```python
from build123d import *

# Parameters (mm, degrees)
SKETCH_1_W            = 118.4
SKETCH_1_H            = 66.4
EXTRUDE_1_DEPTH       = 5.6
SKETCH_5_R            = 3
CUT_EXTRUDE_961_DEPTH = 3
SKETCH_7_W            = 85
SKETCH_7_H            = 58
LCD_DEPTH             = 3.6
SKETCH_13_W           = 73
SKETCH_13_H           = 46
CUT_EXTRUDE_1_DEPTH   = 10
FILLET_2_R            = 5
FILLET_3_R            = 6


with BuildPart() as part:
    # Эскиз1 → Бобышка-Вытянуть1 (new body)
    with BuildSketch(Plane(origin=(0, 0, 0), x_dir=(1, 0, 0), z_dir=(0, 1, 0))):
        with Locations((-2, 0)):
            Rectangle(SKETCH_1_W, SKETCH_1_H)
    extrude(amount=EXTRUDE_1_DEPTH)

    # Эскиз5 → Cut-Extrude 961 (cut)
    with BuildSketch(Plane.XZ):
        with Locations(Location((-56.16, 21.1, 0), (0, 0, 270))):
            Circle(SKETCH_5_R)
        with Locations(Location((-56.16, -21.9, 0), (0, 0, 90))):
            Circle(SKETCH_5_R)
        with Locations(Location((35.96, 22.3, 0), (0, 0, 270))):
            Circle(SKETCH_5_R)
        with Locations(Location((35.96, -18.7, 0), (0, 0, 90))):
            Circle(SKETCH_5_R)
    extrude(amount=-CUT_EXTRUDE_961_DEPTH, mode=Mode.SUBTRACT)

    # Эскиз7 → под LCD (cut)
    with BuildSketch(Plane.XZ):
        with Locations((-10, 0)):
            Rectangle(SKETCH_7_W, SKETCH_7_H)
    extrude(amount=-LCD_DEPTH, mode=Mode.SUBTRACT)

    # Эскиз13 → Вырез-Вытянуть1 (cut)
    with BuildSketch(Plane.XZ.offset(-3.6)):
        with Locations((-10, 0)):
            Rectangle(SKETCH_13_W, SKETCH_13_H)
    extrude(amount=-CUT_EXTRUDE_1_DEPTH, mode=Mode.SUBTRACT)

    # Скругление2
    # the kernel refuses this fillet: 5 mm, written as the material it takes off along each edge
    with BuildSketch(Plane(origin=(-46.5, 5.6, -23), x_dir=(-1, 0, 0), z_dir=(0, 0, 1)), Plane(origin=(26.5, 5.6, 23), x_dir=(1, 0, 0), z_dir=(0, 0, -1))) as fillet_2_piece_1:
        with BuildLine():
            CenterArc((4, 5), FILLET_2_R, 216.869897646, 53.130102354)
            Line((0, 2), (-0.08, 1.94))
            ThreePointArc((-0.08, 1.94), (-0.1, 1), (-0.1, 0))
            Line((-0.1, 0), (0, -0.1))
            Line((0, -0.1), (4, -0.1))
            Line((4, -0.1), (4, 0))
        make_face()
    extrude(amount=46, mode=Mode.SUBTRACT)
    with BuildSketch(Plane(origin=(-46.5, 5.6, 23), x_dir=(0, 0, 1), z_dir=(1, 0, 0)), Plane(origin=(26.5, 5.6, -23), x_dir=(0, 0, -1), z_dir=(-1, 0, 0))) as fillet_2_piece_2:
        with BuildLine():
            CenterArc((4, 5), FILLET_2_R, 216.869897646, 53.130102354)
            Line((0, 2), (-0.08, 1.94))
            ThreePointArc((-0.08, 1.94), (-0.1, 1), (-0.1, 0))
            Line((-0.1, 0), (0, -0.1))
            Line((0, -0.1), (4, -0.1))
            Line((4, -0.1), (4, 0))
        make_face()
    extrude(amount=73, mode=Mode.SUBTRACT)
    with BuildSketch(Plane(origin=(-46.5, 5.6, -33), x_dir=(-1, 0, 0), z_dir=(0, 0, 1))) as fillet_2_piece_3a_section:
        with BuildLine():
            CenterArc((4, 5), FILLET_2_R, 216.869897646, 53.130102354)
            Line((0, 2), (-0.08, 1.94))
            ThreePointArc((-0.08, 1.94), (-0.1, 1), (-0.1, 0))
            Line((-0.1, 0), (0, -0.1))
            Line((0, -0.1), (4, -0.1))
            Line((4, -0.1), (4, 0))
        make_face()
    fillet_2_piece_3a = extrude(amount=56, mode=Mode.PRIVATE)
    fillet_2_piece_3a = split(fillet_2_piece_3a, bisect_by=Plane(origin=(-47.529417057, 5.088057438, -23), z_dir=(0, 0, -1)), keep=Keep.TOP, mode=Mode.PRIVATE)
    with BuildSketch(Plane(origin=(26.5, 5.6, -23), x_dir=(0, 0, -1), z_dir=(-1, 0, 0))) as fillet_2_piece_3b_section:
        with BuildLine():
            CenterArc((4, 5), FILLET_2_R, 216.869897646, 53.130102354)
            Line((0, 2), (-0.08, 1.94))
            ThreePointArc((-0.08, 1.94), (-0.1, 1), (-0.1, 0))
            Line((-0.1, 0), (0, -0.1))
            Line((0, -0.1), (4, -0.1))
            Line((4, -0.1), (4, 0))
        make_face()
    fillet_2_piece_3b = extrude(amount=83, mode=Mode.PRIVATE)
    fillet_2_piece_3b = split(fillet_2_piece_3b, bisect_by=Plane(origin=(-46.5, 5.088057438, -24.029417057), z_dir=(-1, 0, 0)), keep=Keep.TOP, mode=Mode.PRIVATE)
    fillet_2_piece_3 = fillet_2_piece_3a & fillet_2_piece_3b
    add(fillet_2_piece_3, mode=Mode.SUBTRACT)
    with BuildSketch(Plane(origin=(-46.5, 5.6, -23), x_dir=(-1, 0, 0), z_dir=(0, 0, 1))) as fillet_2_piece_4a_section:
        with BuildLine():
            CenterArc((4, 5), FILLET_2_R, 216.869897646, 53.130102354)
            Line((0, 2), (-0.08, 1.94))
            ThreePointArc((-0.08, 1.94), (-0.1, 1), (-0.1, 0))
            Line((-0.1, 0), (0, -0.1))
            Line((0, -0.1), (4, -0.1))
            Line((4, -0.1), (4, 0))
        make_face()
    fillet_2_piece_4a = extrude(amount=56, mode=Mode.PRIVATE)
    fillet_2_piece_4a = split(fillet_2_piece_4a, bisect_by=Plane(origin=(-47.529417057, 5.088057438, 23), z_dir=(0, 0, 1)), keep=Keep.TOP, mode=Mode.PRIVATE)
    with BuildSketch(Plane(origin=(-56.5, 5.6, 23), x_dir=(0, 0, 1), z_dir=(1, 0, 0))) as fillet_2_piece_4b_section:
        with BuildLine():
            CenterArc((4, 5), FILLET_2_R, 216.869897646, 53.130102354)
            Line((0, 2), (-0.08, 1.94))
            ThreePointArc((-0.08, 1.94), (-0.1, 1), (-0.1, 0))
            Line((-0.1, 0), (0, -0.1))
            Line((0, -0.1), (4, -0.1))
            Line((4, -0.1), (4, 0))
        make_face()
    fillet_2_piece_4b = extrude(amount=83, mode=Mode.PRIVATE)
    fillet_2_piece_4b = split(fillet_2_piece_4b, bisect_by=Plane(origin=(-46.5, 5.088057438, 24.029417057), z_dir=(-1, 0, 0)), keep=Keep.TOP, mode=Mode.PRIVATE)
    fillet_2_piece_4 = fillet_2_piece_4a & fillet_2_piece_4b
    add(fillet_2_piece_4, mode=Mode.SUBTRACT)
    with BuildSketch(Plane(origin=(26.5, 5.6, 33), x_dir=(1, 0, 0), z_dir=(0, 0, -1))) as fillet_2_piece_5a_section:
        with BuildLine():
            CenterArc((4, 5), FILLET_2_R, 216.869897646, 53.130102354)
            Line((0, 2), (-0.08, 1.94))
            ThreePointArc((-0.08, 1.94), (-0.1, 1), (-0.1, 0))
            Line((-0.1, 0), (0, -0.1))
            Line((0, -0.1), (4, -0.1))
            Line((4, -0.1), (4, 0))
        make_face()
    fillet_2_piece_5a = extrude(amount=56, mode=Mode.PRIVATE)
    fillet_2_piece_5a = split(fillet_2_piece_5a, bisect_by=Plane(origin=(27.529417057, 5.088057438, 23), z_dir=(0, 0, 1)), keep=Keep.TOP, mode=Mode.PRIVATE)
    with BuildSketch(Plane(origin=(-46.5, 5.6, 23), x_dir=(0, 0, 1), z_dir=(1, 0, 0))) as fillet_2_piece_5b_section:
        with BuildLine():
            CenterArc((4, 5), FILLET_2_R, 216.869897646, 53.130102354)
            Line((0, 2), (-0.08, 1.94))
            ThreePointArc((-0.08, 1.94), (-0.1, 1), (-0.1, 0))
            Line((-0.1, 0), (0, -0.1))
            Line((0, -0.1), (4, -0.1))
            Line((4, -0.1), (4, 0))
        make_face()
    fillet_2_piece_5b = extrude(amount=83, mode=Mode.PRIVATE)
    fillet_2_piece_5b = split(fillet_2_piece_5b, bisect_by=Plane(origin=(26.5, 5.088057438, 24.029417057), z_dir=(1, 0, 0)), keep=Keep.TOP, mode=Mode.PRIVATE)
    fillet_2_piece_5 = fillet_2_piece_5a & fillet_2_piece_5b
    add(fillet_2_piece_5, mode=Mode.SUBTRACT)
    with BuildSketch(Plane(origin=(36.5, 5.6, -23), x_dir=(0, 0, -1), z_dir=(-1, 0, 0))) as fillet_2_piece_6a_section:
        with BuildLine():
            CenterArc((4, 5), FILLET_2_R, 216.869897646, 53.130102354)
            Line((0, 2), (-0.08, 1.94))
            ThreePointArc((-0.08, 1.94), (-0.1, 1), (-0.1, 0))
            Line((-0.1, 0), (0, -0.1))
            Line((0, -0.1), (4, -0.1))
            Line((4, -0.1), (4, 0))
        make_face()
    fillet_2_piece_6a = extrude(amount=83, mode=Mode.PRIVATE)
    fillet_2_piece_6a = split(fillet_2_piece_6a, bisect_by=Plane(origin=(26.5, 5.088057438, -24.029417057), z_dir=(1, 0, 0)), keep=Keep.TOP, mode=Mode.PRIVATE)
    with BuildSketch(Plane(origin=(26.5, 5.6, 23), x_dir=(1, 0, 0), z_dir=(0, 0, -1))) as fillet_2_piece_6b_section:
        with BuildLine():
            CenterArc((4, 5), FILLET_2_R, 216.869897646, 53.130102354)
            Line((0, 2), (-0.08, 1.94))
            ThreePointArc((-0.08, 1.94), (-0.1, 1), (-0.1, 0))
            Line((-0.1, 0), (0, -0.1))
            Line((0, -0.1), (4, -0.1))
            Line((4, -0.1), (4, 0))
        make_face()
    fillet_2_piece_6b = extrude(amount=56, mode=Mode.PRIVATE)
    fillet_2_piece_6b = split(fillet_2_piece_6b, bisect_by=Plane(origin=(27.529417057, 5.088057438, -23), z_dir=(0, 0, -1)), keep=Keep.TOP, mode=Mode.PRIVATE)
    fillet_2_piece_6 = fillet_2_piece_6a & fillet_2_piece_6b
    add(fillet_2_piece_6, mode=Mode.SUBTRACT)

    # Скругление3
    fillet_3_edges = [part.edges().sort_by_distance(p)[0] for p in [
        (-61.2, 2.8, -33.2),
        (57.2, 2.8, -33.2),
        (57.2, 2.8, 33.2),
        (-61.2, 2.8, 33.2),
    ]]
    fillet(fillet_3_edges, radius=FILLET_3_R)


solid = part.part
```
The listing builds one solid part. Answer for the finished solid, in the listing's coordinates (mm). A direction names the side the tool comes from. Round coordinates to 2 decimals unless told otherwise and drop trailing zeros. Write each loop counter-clockwise with the first axis right and the second up, starting at its lowest first coordinate (ties: lowest second). Pieces come first, ordered by that corner, then holes. Notation, with made-up numbers: (80, 3.5) -> (133, 3.5) arc R13 cw to (133, 24.5) -> close; hole circle Ø9 at (46, 80.5). An arc over 180 degrees is marked (long way). Answer as a JSON object with one key per item and string values. Group by question number.
Q1. Section C-C (y = 1) is taken. Write down the section's boundary in (x, z), plus the area to 3 significant figures.
Q2. Straight lines are drawn through the part: line 1 along X through (y, z) = (1.45, -18.7); line 2 along X through (y, z) = (2.2, -21.9); line 3 along Z through (x, y) = (-50, 2.4). For each, find the intervals that lie inside material, in ascending order.
Q3. Which of the six approach directions +Z, -Z, +X, -X, +Y, -Y give full straight-line access (tool end or side, diameter ignored) to faces 1 (the face through (57.2, 3, 0)), 2 (the face through (-10.567, 5.058, 24.735)), 3 (the face through (37.785, 1.479, -21.081))?
Q4. Section D-D (z = 21.1) is taken. Write down the section's boundary in (x, y).
Q5. Section B-B (z = -4) is taken. Write down the section's boundary in (x, y).
Q6. Each of these flat-tipped pins is pushed along its axis until it touches: pin 1 Ø10 at (x, z) = (-42.5, -9.5) entering from +Y; pin 2 Ø5 at (x, z) = (37, 22.5) entering from -Y; pin 3 Ø4 at (x, z) = (-49, 0.5) entering from -Y. Where does it stop, or does it pass through?
Q7. Determine the mould class of faces 4 (the face through (-55.01, 1.48, -19.13)), 5 (the face through (-3, 3, -33.2)), 6 (the face through (55.489, 2.839, 31.396)) for opening direction X: pulls with the +X half, pulls with the -X half, needs draft (parallel to the pull), parting line crosses it, or undercut.
Q8. Section A-A (x = 21) is taken. Write down the section's boundary in (y, z).
Check values:
{
 "1": {"outline": "(-61.2, -27.2) arc R6 ccw to (-55.2, -33.2) -> (51.2, -33.2) arc R6 ccw to (57.2, -27.2) -> (57.2, 27.2) arc R6 ccw to (51.2, 33.2) -> (-55.2, 33.2) arc R6 ccw to (-61.2, 27.2) -> close; hole circle Ø6 at (-56.16, -21.9); hole circle Ø6 at (-56.16, 21.1); hole (-52.5, -29) -> (32.5, -29) -> (32.5, 29) -> (-52.5, 29) -> close; hole circle Ø6 at (35.96, -18.7); hole circle Ø6 at (35.96, 22.3)", "area": "2,790 mm^2"},
 "2": {"line 1": "-61.2 to -52.5, 32.5 to 32.96, 38.96 to 57.2", "line 2": "-61.2 to -59.16, -53.16 to -52.5, 32.5 to 57.2", "line 3": "-33.2 to -29, 29 to 33.2"},
 "3": {"face 1": "+Z, -Z, +X, +Y, -Y", "face 2": "+Y", "face 3": "-Y"},
 "4": {"outline": "(-61.2, 0) -> (-59.16, 0) -> (-59.16, 3) -> (-53.16, 3) -> (-53.16, 0) -> (-52.5, 0) -> (-52.5, 3.6) -> (-46.5, 3.6) arc R5 ccw to (-50.5, 5.6) -> (-61.2, 5.6) -> close; (26.5, 3.6) -> (32.5, 3.6) -> (32.5, 0) -> (33.21, 0) -> (33.21, 3) -> (38.71, 3) -> (38.71, 0) -> (57.2, 0) -> (57.2, 5.6) -> (30.5, 5.6) arc R5 ccw to start"},
 "5": {"outline": "(-61.2, 0) -> (-52.5, 0) -> (-52.5, 3.6) -> (-46.5, 3.6) arc R5 ccw to (-50.5, 5.6) -> (-61.2, 5.6) -> close; (26.5, 3.6) -> (32.5, 3.6) -> (32.5, 0) -> (57.2, 0) -> (57.2, 5.6) -> (30.5, 5.6) arc R5 ccw to start"},
 "6": {"pin 1": "y = 4.6", "pin 2": "y = 0", "pin 3": "y = 3.6"},
 "7": {"face 4": "undercut", "face 5": "needs draft", "face 6": "pulls with the +X half"},
 "8": {"outline": "(0, -33.2) -> (5.6, -33.2) -> (5.6, -27) arc R5 ccw to (3.6, -23) -> (3.6, -29) -> (0, -29) -> close; (0, 29) -> (3.6, 29) -> (3.6, 23) arc R5 ccw to (5.6, 27) -> (5.6, 33.2) -> (0, 33.2) -> close"}
}
